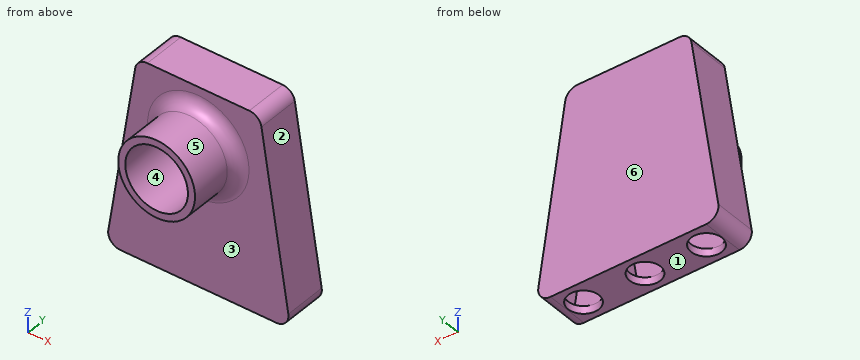
```python
from build123d import *

# Parameters (mm, degrees)
F1_DEPTH  = 2.54
F3_DEPTH  = 6.35
F5_W      = 2.54
F5_H      = 25.4
F6_DEPTH  = 6.35
F7_W      = 2.54
F7_H      = 25.4
F8_DEPTH  = 6.35
F9_R      = 6.35
F10_DEPTH = 25.4
F11_R     = 15.875
F12_DEPTH = 22.225
F13_R     = 12.954
F14_DEPTH = 31.75
F15_R     = 5.08


with BuildPart() as f1:
    # F0 (on Front) → F1 (new body)
    with BuildSketch(Plane.XZ):
        Polygon((25.4, 0), (-25.4, 0), (-38.1, -81.5672268745), (38.1, -81.5672268745), align=None)
    extrude(amount=F1_DEPTH)

    # F2 (on face) → F3 (join)
    with BuildSketch(Plane.XZ.offset(2.54)):
        Polygon((-38.1, -81.5672268745), (38.1, -81.5672268745), (25.4, 0), (-25.4, 0), align=None)
        Polygon((20.1079053095, -3.175), (22.6810924375, -3.175), (34.3923987784, -78.3922268745), (10.4823719593, -78.3922268745), (7.9091848312, -78.3922268745), (-7.9091848312, -78.3922268745), (-10.4823719593, -78.3922268745), (-34.3923987784, -78.3922268745), (-22.6810924375, -3.175), (-20.1079053095, -3.175), align=None, mode=Mode.SUBTRACT)
        Polygon((-7.9091848312, -78.3922268745), (-20.1079053095, -3.175), (-22.6810924375, -3.175), (-10.4823719593, -78.3922268745), align=None)
        Polygon((10.4823719593, -78.3922268745), (22.6810924375, -3.175), (20.1079053095, -3.175), (7.9091848312, -78.3922268745), align=None)
    extrude(amount=F3_DEPTH)

    # F4: F1 across face


with BuildPart() as f1_1:
    add(f1.part)
    add(f1.part.mirror(Plane(origin=(0, -8.89, -43.1700299624), x_dir=(1, 0, 0), z_dir=(0, -1, 0))))

    # F5 (on face) → F6 (cut)
    with BuildSketch(Plane(origin=(22.6015407656, 0, -3.665515064), x_dir=(0, 1, 0), z_dir=(0.9871027149, 0, -0.1600881953))):
        with Locations((-3.81, -24.3075852952)):
            Rectangle(F5_W, F5_H)
    extrude(amount=-F6_DEPTH, mode=Mode.SUBTRACT)

    # F7 (on face) → F8 (cut)
    with BuildSketch(Plane(origin=(-20.0942998698, 0, -3.258891048), x_dir=(0, 1, 0), z_dir=(0.9871027149, 0, 0.1600881953))):
        with Locations((-3.81, -25.4971986666)):
            Rectangle(F7_W, F7_H)
    extrude(amount=-F8_DEPTH, mode=Mode.SUBTRACT)

    # F9 (on face) → F10 (cut)
    with BuildSketch(Plane(origin=(0, 0, -81.5672268745), x_dir=(1, 0, 0), z_dir=(0, 0, -1))):
        with Locations((-25.4, 8.89)):
            Circle(F9_R)
        with Locations((0, 8.89)):
            Circle(F9_R)
        with Locations((25.4, 8.89)):
            Circle(F9_R)
    extrude(amount=-F10_DEPTH, mode=Mode.SUBTRACT)

    # F11 (on face) → F12 (join)
    with BuildSketch(Plane.XZ.offset(17.78)):
        with Locations((0, -24.4172268745)):
            Circle(F11_R)
    extrude(amount=F12_DEPTH)

    # F13 (on face) → F14 (cut)
    with BuildSketch(Plane.XZ.offset(40.005)):
        with Locations((0, -24.4172268745)):
            Circle(F13_R)
    extrude(amount=-F14_DEPTH, mode=Mode.SUBTRACT)

    # F15
    f15_edges = [f1_1.edges().sort_by_distance(p)[0] for p in [
        (-15.875, -17.78, -24.417227),
        (-38.1, -8.89, -81.567227),
        (38.1, -8.89, -81.567227),
        (25.4, -8.89, 0),
        (-25.4, -8.89, 0),
    ]]
    fillet(f15_edges, radius=F15_R)


solid = f1_1.part
```
The listing builds one solid part. Answer for the finished solid, in the listing's coordinates (mm). Face numbers are marked on the shaded views. A direction names the side the tool comes from. Round coordinates to 2 decimals unless told otherwise and drop trailing zeros. Loops run counter-clockwise (first coordinate to the right, second up) from the corner with the lowest first, then second, coordinate; pieces in that order, holes last.
1) For the marked faces 5 and 6, determine the directions among +Z, -Z, +X, -X, +Y, -Y from which every point of the face is accessible in a straight line to the end or side of a thin tool.
Outcome:
face 5: -Y
face 6: +Z, -Z, +X, -X, +Y
2) Consider line 1 (Y direction, x = 20, z = -41.5); line 2 (X direction, y = -6, z = -49); line 3 (Y direction, x = 22, z = -4). Determine where each line is inside the solid, lowest interval first.
Outcome:
line 1: y = -17.78 to -15.24, -2.54 to 0
line 2: x = -33.03 to -29.82, -15.25 to -12.68, 12.68 to 15.25, 29.82 to 33.03
line 3: y = -17.78 to 0
3) A cutting plane is placed at D-D on z = -52. Determine the outline of the cut face in (x, y).
Outcome:
outline: (-33.5, -17.78) - (33.5, -17.78) - (33.5, 0) - (-33.5, 0) - close; hole (-30.28, -15.24) - (-14.76, -15.24) - (-14.76, -2.54) - (-30.28, -2.54) - close; hole (-12.19, -15.24) - (12.19, -15.24) - (12.19, -2.54) - (-12.19, -2.54) - close; hole (14.76, -15.24) - (30.28, -15.24) - (30.28, -2.54) - (14.76, -2.54) - close
4) For a pull along Z with two mould halves and no side action, classify the marked faces 1, 2, 3 and 4 as released by +Z, released by -Z, zero draft, split by the parting line, or undercut.
Outcome:
face 1: released by -Z
face 2: released by +Z
face 3: zero draft
face 4: undercut
5) A cutting plane is placed at A-A on z = -67.5. Determine the outline of the cut face in (x, y).
Outcome:
outline: (-35.91, -17.78) - (35.91, -17.78) - (35.91, 0) - (-35.91, 0) - close; hole (-32.7, -15.24) - (-12.25, -15.24) - (-12.25, -2.54) - (-32.7, -2.54) - close; hole (-9.68, -15.24) - (9.68, -15.24) - (9.68, -2.54) - (-9.68, -2.54) - close; hole (12.25, -15.24) - (32.7, -15.24) - (32.7, -2.54) - (12.25, -2.54) - close
6) A cutting plane is placed at B-B on y = -30. Determine the outline of the cut face in (x, z) (3 decimals), plus the area to 3 significant figures.
Outcome:
outline: circle Ø31.75 at (0, -24.417); hole circle Ø25.908 at (0, -24.417)
area: 265 mm2
7) Given P1, Ø12, axis at y = -4, z = -27, coming from the -X side; P2, Ø1.5, axis at x = -15, z = -34.5, coming from the -Y side; P3, Ø10, axis at x = -11, z = -60, coming from the -Y side; P4, Ø8, axis at x = -29, z = -21, coming from the +Y side, each flat-ended and moving along its own axis, determine where each tip first touches the part or whether it passes through.
Outcome:
P1: stops at x = -30.54
P2: stops at y = -19.31
P3: stops at y = -17.78
P4: stops at y = 0
